The model under review builds one solid part; all positions refer to its coordinate system, in mm. Face numbers are marked on the shaded views. A direction names the side the tool comes from. Coordinates: 2 decimals unless noted, no trailing zeros. Loops run counter-clockwise (first coordinate to the right, second up) from the corner with the lowest first, then second, coordinate; pieces in that order, holes last. Notation, with made-up numbers: M 38,12.5 L 84,12.5 A33 cw 84,40.5 Z; hole C 52.5,0.25 d10. An arc over 180 degrees is marked long. Use CSV: the item, a comma, the result in double quotes. Start each with the question number.
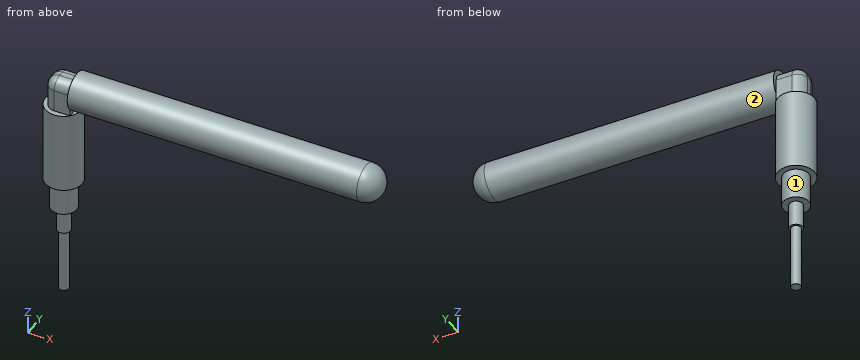
from build123d import *

# Parameters (mm, degrees)
SKETCH1_R           = 4.572
BOSS_EXTRUDE1_DEPTH = 20.32
SKETCH2_R           = 3.175
BOSS_EXTRUDE2_DEPTH = 7.62
SKETCH3_R           = 1.651
BOSS_EXTRUDE3_DEPTH = 6.35
SKETCH4_R           = 1.2065
BOSS_EXTRUDE4_DEPTH = 16.002
SKETCH8_W           = 6.465784408
SKETCH8_H           = 6.465784408
BOSS_EXTRUDE5_DEPTH = 8.0518
SKETCH10_R          = 4.572
BOSS_EXTRUDE6_DEPTH = 71.628
DOME4_FACE_RADIUS   = 4.572
DOME4_HEIGHT        = 4.572
FILLET1_R           = 2.54


with BuildPart() as part:
    # Sketch1 → Boss-Extrude1 (new body)
    with BuildSketch(Plane.XY):
        Circle(SKETCH1_R)
    extrude(amount=BOSS_EXTRUDE1_DEPTH)

    # Sketch2 → Boss-Extrude2 (add)
    with BuildSketch(Plane(origin=(0, 0, 0), x_dir=(-1, 0, 0), z_dir=(0, 0, -1))):
        Circle(SKETCH2_R)
    extrude(amount=BOSS_EXTRUDE2_DEPTH)

    # Sketch3 → Boss-Extrude3 (add)
    with BuildSketch(Plane(origin=(0, 0, -7.62), x_dir=(-1, 0, 0), z_dir=(0, 0, -1))):
        Circle(SKETCH3_R)
    extrude(amount=BOSS_EXTRUDE3_DEPTH)

    # Sketch4 → Boss-Extrude4 (add)
    with BuildSketch(Plane(origin=(0, 0, -13.97), x_dir=(-1, 0, 0), z_dir=(0, 0, -1))):
        Circle(SKETCH4_R)
    extrude(amount=BOSS_EXTRUDE4_DEPTH)

    # Sketch8 → Boss-Extrude5 (add)
    with BuildSketch(Plane.XY.offset(20.32)):
        Rectangle(SKETCH8_W, SKETCH8_H)
    extrude(amount=BOSS_EXTRUDE5_DEPTH)

    # Sketch10 → Boss-Extrude6 (add)
    with BuildSketch(Plane(origin=(3.232892204, 0, 0), x_dir=(0, 0, -1), z_dir=(1, 0, 0))):
        with Locations((-25.2349, 0)):
            Circle(SKETCH10_R)
    extrude(amount=BOSS_EXTRUDE6_DEPTH)

    # Dome4: a dome of height H over a round flat face of radius A is a cap of a sphere of radius (A * A + H * H) / (2 * H)
    dome4_r = (DOME4_FACE_RADIUS * DOME4_FACE_RADIUS + DOME4_HEIGHT * DOME4_HEIGHT) / (2 * DOME4_HEIGHT)
    dome4_base = Plane((74.860892204, 0, 25.2349), z_dir=(1, 0, 0))
    with Locations(dome4_base.offset(DOME4_HEIGHT - dome4_r)):
        dome4_ball = Sphere(dome4_r, mode=Mode.PRIVATE)
    add(split(dome4_ball, bisect_by=dome4_base, keep=Keep.TOP, mode=Mode.PRIVATE))

    # Fillet1
    fillet1_edges = [part.edges().sort_by_distance(p)[0] for p in [
        (-3.232892204, 3.232892204, 24.3459),
        (-3.232892204, -3.232892204, 24.3459),
        (0, 3.232892204, 28.3718),
        (-3.232892204, 0, 28.3718),
        (0, -3.232892204, 28.3718),
    ]]
    fillet(fillet1_edges, radius=FILLET1_R)


solid = part.part
1. Add section C-C (z = -6.5). Write out the cut boundary in (x, y) (3 decimals).
2. To check wall thickness, follow line 1 along Y through (x, z) = (57.5, 22); line 2 along X through (y, z) = (-0.25, 15); line 3 along Z through (x, y) = (60, -4). State the ranges of each line that lie inside material, in increasing order.
3. For the marked faces 1 and 2, list the 3-axis set-ups (+Z, -Z, +X, -X, +Y, -Y) from which the entire face can be reached by the end or side of a thin tool; tool diameter is ignored.
4. Insertion check: pin 1 Ø4 at (y, z) = (-1.5, 27) entering from -X; pin 2 Ø1.5 at (y, z) = (0.5, -20.5) entering from +X; pin 3 Ø2 at (x, y) = (23, -2) entering from +Z. Each pin has a flat end and moves straight along its axis. Give the tip position at first contact, or say it passes through.
5. Add section A-A (z = 23). Write out the cut boundary in (x, y), plus the area to 3 significant figures.
6. Add section B-B (x = 37.5). Write out the cut boundary in (y, z).
Solved:
1,outline,"C 0,0 d6.35"
2,line 1,"y = -3.23 to 3.23"
2,line 2,"x = -4.57 to 4.57"
2,line 3,"z = 23.02 to 27.45"
3,face 1,"-Z"
3,face 2,"+X"
4,pin 1,"stops at x = -3.23"
4,pin 2,"stops at x = 1.21"
4,pin 3,"stops at z = 29.7"
5,outline,"M -3.23,-0.69 A2.54 ccw -0.69,-3.23 L 3.23,-3.23 L 3.23,-3.99 L 74.86,-3.99 A3.99 ccw 74.86,3.99 L 3.23,3.99 L 3.23,3.23 L -0.69,3.23 A2.54 ccw -3.23,0.69 Z"
5,area,"635 mm^2"
6,outline,"C 0,25.23 d9.14"
